Design review of the part built by this model. Coordinates are the model's own, in mm. A direction names the side the tool comes from. Give positions to 0.01 mm unless a question says otherwise; leave off trailing zeros. Write each loop counter-clockwise with the first axis right and the second up, starting at its lowest first coordinate (ties: lowest second). Pieces come first, ordered by that corner, then holes. Notation, with made-up numbers: M 45,-22 L 97,-22 A25 ccw 97,14 Z; hole C 2.5,13 d9. An arc over 180 degrees is marked long. Use a Markdown table: item, result. Add a question column.
```python
from build123d import *

# Parameters (mm, degrees)
DIAMETRE_TETE_R     = 27
HAUTEUR_TETE_DEPTH  = 36
CONGE_R             = 3
DIAMETRE_R          = 18
LONGUEUR_DEPTH      = 170
HAUTEUR_6PANS_DEPTH = 18
CHANFREIN_SIZE      = 3


with BuildPart() as part:
    # DIAMETRE_TETE → HAUTEUR_TETE (new body)
    with BuildSketch(Plane(origin=(0, 0, 0), x_dir=(1, 0, 0), z_dir=(0, 1, 0))):
        with Locations(Location((0, 0, 0), (0, 0, 270))):
            Circle(DIAMETRE_TETE_R)
    extrude(amount=HAUTEUR_TETE_DEPTH)

    # CONGE
    conge_edges = [part.edges().sort_by_distance(p)[0] for p in [
        (0, 36, -27),
    ]]
    fillet(conge_edges, radius=CONGE_R)

    # DIAMETRE → LONGUEUR (add)
    with BuildSketch(Plane.XZ):
        with Locations(Location((0, 0, 0), (0, 0, 270))):
            Circle(DIAMETRE_R)
    extrude(amount=LONGUEUR_DEPTH)

    # LARGEUR_6PANS → HAUTEUR_6PANS (cut)
    with BuildSketch(Plane(origin=(0, 36, 0), x_dir=(1, 0, 0), z_dir=(0, 1, 0))):
        Polygon((8.142672131, 13.292738265), (-7.440512958, 13.698130052), (-15.583185088, 0.405391788), (-8.142672131, -13.292738265), (7.440512958, -13.698130052), (15.583185088, -0.405391788), align=None)
    extrude(amount=-HAUTEUR_6PANS_DEPTH, mode=Mode.SUBTRACT)

    # CHANFREIN
    chanfrein_edges = [part.edges().sort_by_distance(p)[0] for p in [
        (0, -170, 18),
    ]]
    chamfer(chanfrein_edges, length=CHANFREIN_SIZE)


solid = part.part
```
(1) Wall thickness on L1, parallel to Z at x = 1, y = -41; L2, parallel to Y at x = -19, z = -10; L3, parallel to X at y = 7.5, z = -1.5: over which ranges is each line inside the solid? List them lowest first.
(2) The part is to be moulded in two halves that separate along Z. For faces 4 (the flat face through (-18, 0, 6)), 5 (the cylindrical face through (-26.36, 16.27, -5.85)), 6 (the flat face through (-11.455, 27.126, -7.145)), say which applies: released by +Z, released by -Z, zero draft, split by the parting line, or undercut.
(3) Add section A-A on x = 0. Give the boundary of the cut face in (y, z), then the cut area to 3 significant figures.
(4) Add section B-B on y = -84.5. Give the boundary of the cut face in (x, z).
(5) Machinability: for faces 1 (the flat face through (-10.3, 36, 10.3)), 2 (the cylindrical face through (5.407, -82.331, -17.169)), 3 (the flat face through (11.455, 27.126, 7.145)), which of the approach directions +Z, -Z, +X, -X, +Y, -Y give a long, thin tool a straight path to every point of the face, cutting with its end or side? Answer none if there is none.
(6) For pin 1 (10 mm diameter, centred on x = 0.5, y = -13, fed in from -Z); pin 2 (4 mm diameter, centred on x = 21, y = -123, fed in from -Z); pin 3 (12 mm diameter, centred on x = -20, y = -7, fed in from -Z); pin 4 (12 mm diameter, centred on x = -3, z = -5, fed in from +Y), all flat-tipped, find the tip position at first contact; note any pin that passes through.
From the geometry:
| question | item | result |
|---|---|---|
| 1 | L1 | z = -17.97 to 17.97 |
| 1 | L2 | y = 0 to 36 |
| 1 | L3 | x = -26.96 to 26.96 |
| 2 | face 4 | zero draft |
| 2 | face 5 | split by the parting line |
| 2 | face 6 | undercut |
| 3 | outline | M -170,-15 L -167,-18 L 0,-18 L 0,-27 L 33,-27 A3 ccw 36,-24 L 36,-13.5 L 18,-13.5 L 18,13.5 L 36,13.5 L 36,24 A3 ccw 33,27 L 0,27 L 0,18 L -167,18 L -170,15 Z |
| 3 | area | 7,560 mm^2 |
| 4 | outline | C 0,0 d36 |
| 5 | face 1 | +Z, -Z, +X, -X, +Y |
| 5 | face 2 | -Y |
| 5 | face 3 | +Y |
| 6 | pin 1 | stops at z = -18 |
| 6 | pin 2 | passes through |
| 6 | pin 3 | stops at z = -11.31 |
| 6 | pin 4 | stops at y = 18 |
